Geometry check sheet. Reference: the model listing, model coordinates, mm. Face numbers are marked on the shaded views. A direction names the side the tool comes from. Give positions to 0.01 mm unless a question says otherwise; leave off trailing zeros. Write each loop counter-clockwise with the first axis right and the second up, starting at its lowest first coordinate (ties: lowest second). Pieces come first, ordered by that corner, then holes. Notation, with made-up numbers: (51, -27) -> (78, -27) arc R22 ccw to (78, -10) -> close; hole circle Ø6 at (46, 55). An arc over 180 degrees is marked (long way). One line per item, written item: value.
from build123d import *

# Parameters (mm, degrees)
SKETCH1_R           = 1.27
BOSS_EXTRUDE1_DEPTH = 15.24
BIG_FILL_R          = 6.35
FILLET1_R           = 2.54


with BuildPart() as part:
    # Sketch1 → Boss-Extrude1 (new body)
    with BuildSketch(Plane.XY):
        Polygon((0, 0), (-14.108343909, 0), (-18.190770029, 4.082426119), (-22.399065773, 4.082426119), (-22.068202315, 0), (-28.595630403, 0), (-28.595630403, 8.89), (-0.090256121, 8.89), (1.705795103, 10.686051224), (1.705795103, 36.086051224), (-7.919873827, 49.670016208), (-3.692519109, 52.665541963), (8.055795103, 36.086051224), (8.055795103, 8.055795103), align=None)
        with Locations(Location((-0.045128061, 4.445, 0), (0, 0, 180))):
            Circle(SKETCH1_R, mode=Mode.SUBTRACT)
        with Locations(Location((4.880795103, 31.006051224, 0), (0, 0, 180))):
            Circle(SKETCH1_R, mode=Mode.SUBTRACT)
    extrude(amount=BOSS_EXTRUDE1_DEPTH)

    # big_fill
    big_fill_edges = [part.edges().sort_by_distance(p)[0] for p in [
        (0, 0, 7.62),
        (8.055795103, 36.086051224, 7.62),
        (8.055795103, 8.055795103, 7.62),
    ]]
    fillet(big_fill_edges, radius=BIG_FILL_R)

    # Fillet1
    fillet1_edges = [part.edges().sort_by_distance(p)[0] for p in [
        (-28.595630403, 0, 7.62),
        (-28.595630403, 8.89, 7.62),
        (-7.919873827, 49.670016208, 7.62),
        (-3.692519109, 52.665541963, 7.62),
    ]]
    fillet(fillet1_edges, radius=FILLET1_R)


solid = part.part
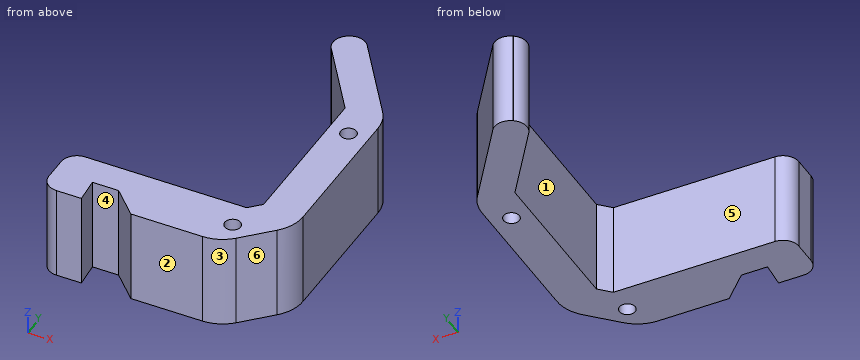
1) Sectioned sample at A-A on y = 5. Record the cut outline in (x, z).
Verdict:
outline: (-28.6, 0) -> (-1.19, 0) -> (-1.19, 15.24) -> (-28.6, 15.24) -> close; (1.1, 0) -> (5, 0) -> (5, 15.24) -> (1.1, 15.24) -> close
2) Depth check by flat-ended pin: pin 1 Ø2 at (x, z) = (-10, 13.5) entering from +Y; pin 2 Ø3 at (x, z) = (-18, 7.5) entering from -Y; pin 3 Ø8 at (x, z) = (1.5, 13) entering from +Y. Enter the tip coordinate at first touch or a pass-through.
Verdict:
pin 1: y = 8.89
pin 2: y = 2.39
pin 3: y = 50.92
3) Mould release check, pull along X, two halves, no side actions. Record for the marked faces 1, 2, 3 and 4: released by +X, released by -X, zero draft, split by the parting line, or undercut.
Verdict:
face 1: released by -X
face 2: zero draft
face 3: released by +X
face 4: undercut
4) Scan lines: probe 1 along Y at (x, z) = (-1, 8.5); probe 2 along Y at (x, z) = (1, 5.75); probe 3 along X at (y, z) = (13, 8.5). Record each from-to range of solid material in increasing order.
Verdict:
probe 1: 0.21 to 3.61, 5.28 to 8.89, 39.9 to 48.87
probe 2: 1.14 to 3.72, 5.17 to 9.98, 37.08 to 46.04
probe 3: 1.71 to 8.06
5) Sectioned sample at B-B on x = 5. Record the cut outline in (y, z), plus the area to 3 significant figures.
Verdict:
outline: (5, 0) -> (29.74, 0) -> (29.74, 15.24) -> (5, 15.24) -> close; (32.27, 0) -> (40.4, 0) -> (40.4, 15.24) -> (32.27, 15.24) -> close
area: 501 mm^2
6) Sectioned sample at C-C on z = 9. Record the cut outline in (x, y) (3 decimals).
Verdict:
outline: (-28.596, 2.54) arc R2.54 ccw to (-26.056, 0) -> (-22.068, 0) -> (-22.399, 4.082) -> (-18.191, 4.082) -> (-14.108, 0) -> (-2.63, 0) arc R6.35 ccw to (1.86, 1.86) -> (6.196, 6.196) arc R6.35 ccw to (8.056, 10.686) -> (8.056, 34.064) arc R6.35 ccw to (6.887, 37.736) -> (-2.224, 50.593) arc R2.54 ccw to (-5.765, 51.197) -> (-5.847, 51.139) arc R2.54 ccw to (-6.451, 47.598) -> (1.706, 36.086) -> (1.706, 10.686) -> (-0.09, 8.89) -> (-26.056, 8.89) arc R2.54 ccw to (-28.596, 6.35) -> close; hole circle Ø2.54 at (-0.045, 4.445); hole circle Ø2.54 at (4.881, 31.006)
7) Sectioned sample at D-D on x = -25.5. Record the cut outline in (y, z).
Verdict:
outline: (0, 0) -> (8.89, 0) -> (8.89, 15.24) -> (0, 15.24) -> close
8) Tool access check on the marked faces 5 and 6. Record the directions out of +Z, -Z, +X, -X, +Y, -Y that give a thin tool (end or side, any length) a straight path to the whole face; none if there is none.
Verdict:
face 5: +Z, -Z, -X
face 6: +Z, -Z, +X, -Y
